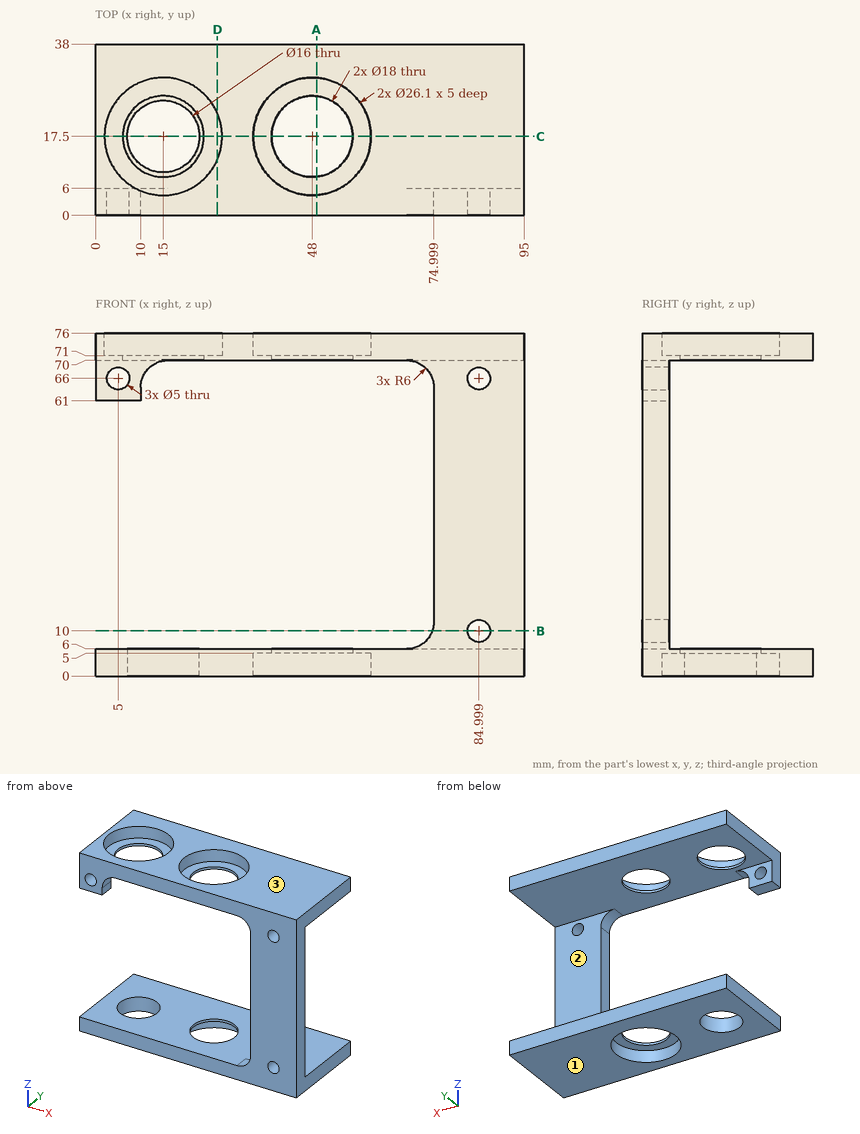
Could you check a few things on this drawing? It's one solid part, dimensions in mm from its lowest x, y, z. Give positions to 0.01 mm unless a question says otherwise; leave off trailing zeros. Write each loop counter-clockwise with the first axis right and the second up, starting at its lowest first coordinate (ties: lowest second). Pieces come first, ordered by that corner, then holes.
(1) If I drill on L1, parallel to Y at x = 48, z = 5.7; L2, parallel to Z at x = 81, y = 18; L3, parallel to X at y = 1.9, z = 66 (1 decimal), over which ranges is the centre line in solid material (lowest first)?
Output values:
L1: y = 0 to 8.5, 26.5 to 38
L2: z = 0 to 6, 70 to 76
L3: x = 0 to 2.5, 7.5 to 10.3, 74.7 to 82.5, 87.5 to 95
(2) Imagine slicing it at C-C, the plane y = 17.5. Count the separate pieces of the cut face and the enclosed holes in it.
Output values:
separate pieces: 6
enclosed holes: 0
(3) Will these pins go through, and if not, where does the flat tip stop? pin 1 (4.5 mm diameter, centred on x = 85, z = 10, fed in from -Y); pin 2 (8 mm diameter, centred on x = 45.5, y = 22.5, fed in from +Z); pin 3 (6.5 mm diameter, centred on y = 3.5, z = 27.5, fed in from -X).
Output values:
pin 1: passes through
pin 2: stops at z = 71
pin 3: stops at x = 75
(4) Imagine slicing it at B-B, the plane z = 10. Write out the boundary of the cut face in (x, y) (1 decimal).
Output values:
outline: (74.7, 0) - (82.5, 0) - (82.5, 6) - (74.7, 6) - close; (87.5, 0) - (95, 0) - (95, 6) - (87.5, 6) - close
(5) Imagine slicing it at A-A, the plane x = 49. Write out the boundary of the cut face in (y, z) (1 decimal).
Output values:
outline: (0, 0) - (4.5, 0) - (4.5, 5) - (8.6, 5) - (8.6, 6) - (0, 6) - close; (0, 70) - (8.6, 70) - (8.6, 71) - (4.5, 71) - (4.5, 76) - (0, 76) - close; (26.4, 5) - (30.5, 5) - (30.5, 0) - (38, 0) - (38, 6) - (26.4, 6) - close; (26.4, 70) - (38, 70) - (38, 76) - (30.5, 76) - (30.5, 71) - (26.4, 71) - close
(6) Thinking about a two-plate mould opening in Z: for the marked faces 1, 2 and 3, which applies, pulls with the +Z half, pulls with the -Z half, needs draft (parallel to the pull), parting line crosses it, or undercut?
Output values:
face 1: pulls with the -Z half
face 2: undercut
face 3: pulls with the +Z half
(7) Imagine slicing it at D-D, the plane x = 27. Write out the boundary of the cut face in (y, z).
Output values:
outline: (0, 0) - (38, 0) - (38, 6) - (0, 6) - close; (0, 70) - (38, 70) - (38, 76) - (22.63, 76) - (22.63, 71) - (12.37, 71) - (12.37, 76) - (0, 76) - close
